Build history of the part. All positions in model axes, mm. A direction names the side the tool comes from. Give positions to 0.01 mm unless a question says otherwise; leave off trailing zeros. Write each loop counter-clockwise with the first axis right and the second up, starting at its lowest first coordinate (ties: lowest second). Pieces come first, ordered by that corner, then holes. Notation, with made-up numbers: (-11.5, 55) -> (25.5, 55) arc R19 cw to (25.5, 90) -> close; hole circle Ø5 at (-28, 74.5). An arc over 180 degrees is marked (long way). Put each result on its own line as item: value.
from build123d import *

# Parameters (mm, degrees)
SKETCH3_R           = 2.15
BOSS_EXTRUDE1_DEPTH = 5
SKETCH4_R           = 36
BOSS_EXTRUDE2_DEPTH = 41
SKETCH5_R           = 9.55
CUT_EXTRUDE1_DEPTH  = 6.2
SKETCH6_R           = 32
CUT_EXTRUDE2_DEPTH  = 36
SKETCH8_R           = 6
CUT_EXTRUDE3_DEPTH  = 76.060242472


with BuildPart() as part:
    # Sketch3 → Boss-Extrude1 (new body)
    with BuildSketch(Plane(origin=(0, 0, 0), x_dir=(1, 0, 0), z_dir=(0, 1, 0))):
        with BuildLine():
            Line((-35, 45), (35, 45))
            ThreePointArc((35, 45), (42.071067812, 42.071067812), (45, 35))
            Line((45, 35), (45, -35))
            ThreePointArc((45, -35), (42.071067812, -42.071067812), (35, -45))
            Line((35, -45), (-35, -45))
            ThreePointArc((-35, -45), (-42.071067812, -42.071067812), (-45, -35))
            Line((-45, -35), (-45, 35))
            ThreePointArc((-45, 35), (-42.071067812, 42.071067812), (-35, 45))
        make_face()
        with Locations(Location((-36, 36, 0), (0, 0, 270))):
            Circle(SKETCH3_R, mode=Mode.SUBTRACT)
        with Locations(Location((36, 36, 0), (0, 0, 270))):
            Circle(SKETCH3_R, mode=Mode.SUBTRACT)
        with Locations(Location((36, -36, 0), (0, 0, 270))):
            Circle(SKETCH3_R, mode=Mode.SUBTRACT)
        with Locations(Location((-36, -36, 0), (0, 0, 270))):
            Circle(SKETCH3_R, mode=Mode.SUBTRACT)
    extrude(amount=BOSS_EXTRUDE1_DEPTH)

    # Sketch4 → Boss-Extrude2 (add)
    with BuildSketch(Plane(origin=(0, 5, 0), x_dir=(1, 0, 0), z_dir=(0, 1, 0))):
        with Locations(Location((0, 0, 0), (0, 0, 270))):
            Circle(SKETCH4_R)
    extrude(amount=BOSS_EXTRUDE2_DEPTH)

    # Sketch5 → Cut-Extrude1 (cut)
    with BuildSketch(Plane(origin=(0, 46, 0), x_dir=(1, 0, 0), z_dir=(0, 1, 0))):
        with Locations(Location((0, 0, 0), (0, 0, 270))):
            Circle(SKETCH5_R)
    extrude(amount=-CUT_EXTRUDE1_DEPTH, mode=Mode.SUBTRACT)

    # Sketch6 → Cut-Extrude2 (cut)
    with BuildSketch(Plane.XZ):
        with Locations(Location((0, 0, 0), (0, 0, 270))):
            Circle(SKETCH6_R)
    extrude(amount=-CUT_EXTRUDE2_DEPTH, mode=Mode.SUBTRACT)

    # Sketch8 → Cut-Extrude3 (cut, through all)
    with BuildSketch(Plane(origin=(0, 39.8, 0), x_dir=(1, 0, 0), z_dir=(0, 1, 0))):
        with Locations(Location((0, 0, 0), (0, 0, 270))):
            Circle(SKETCH8_R)
    extrude(amount=-CUT_EXTRUDE3_DEPTH, mode=Mode.SUBTRACT)


solid = part.part
1) Pull direction Z, two halves, no side cores. Call faces 4 (the flat face through (31, 5, -21)), 5 (the flat face through (-6.2, 39.8, -0.1)), 6 (the flat face through (0, 2, -45)), 7 (the cylindrical face through (-41.99, 2.46, 42.15)): released by +Z, released by -Z, zero draft, split by the parting line, or undercut.
Filled sheet:
face 4: zero draft
face 5: undercut
face 6: released by -Z
face 7: released by +Z
2) Wall check: L1, parallel to X at y = 3, z = 36; L2, parallel to X at y = 16, z = 0; L3, parallel to Y at x = 19.5, z = -13. Give the ranges that are in metal, low to high.
Filled sheet:
L1: -44.95 to -38.15, -33.85 to 33.85, 38.15 to 44.95
L2: -36 to -32, 32 to 36
L3: 36 to 46
3) Slice it at D-D (y = 7.5). Write the cut outline in (x, z).
Filled sheet:
outline: circle Ø72 at (0, 0); hole circle Ø64 at (0, 0)
4) Slice it at C-C (x = -23.5). Write the cut outline in (y, z), plus the area to 3 significant figures.
Filled sheet:
outline: (0, -45) -> (5, -45) -> (5, -27.27) -> (46, -27.27) -> (46, 27.27) -> (5, 27.27) -> (5, 45) -> (0, 45) -> (0, 21.72) -> (36, 21.72) -> (36, -21.72) -> (0, -21.72) -> close
area: 1,120 mm2
5) Slice it at B-B (z = 0). Write the cut outline in (x, y), plus the area to 3 significant figures.
Filled sheet:
outline: (-45, 0) -> (-32, 0) -> (-32, 36) -> (-6, 36) -> (-6, 39.8) -> (-9.55, 39.8) -> (-9.55, 46) -> (-36, 46) -> (-36, 5) -> (-45, 5) -> close; (6, 36) -> (32, 36) -> (32, 0) -> (45, 0) -> (45, 5) -> (36, 5) -> (36, 46) -> (9.55, 46) -> (9.55, 39.8) -> (6, 39.8) -> close
area: 934 mm2
6) Slice it at A-A (x = 0). Write the cut outline in (y, z), plus the area to 3 significant figures.
Filled sheet:
outline: (0, -45) -> (5, -45) -> (5, -36) -> (46, -36) -> (46, -9.55) -> (39.8, -9.55) -> (39.8, -6) -> (36, -6) -> (36, -32) -> (0, -32) -> close; (0, 32) -> (36, 32) -> (36, 6) -> (39.8, 6) -> (39.8, 9.55) -> (46, 9.55) -> (46, 36) -> (5, 36) -> (5, 45) -> (0, 45) -> close
area: 934 mm2
7) Pin check, flat tips, straight feed: pin 1 (19 mm diameter, centred on x = -15.5, z = 14, fed in from -Y); pin 2 (6 mm diameter, centred on x = -11.5, y = 12, fed in from +Z); pin 3 (2 mm diameter, centred on x = -28.5, y = 29, fed in from -Z). Stop position of each tip, or through.
Filled sheet:
pin 1: y = 36
pin 2: z = 34.98
pin 3: z = -23.23
8) Tool access for faces 1 (the flat face through (-45, 2, 0)), 2 (the cylindrical face through (-31.24, 17.75, 6.94)), 3 (the cylindrical face through (2.9, 42.9, 9.1)): list every direction of +Z, -Z, +X, -X, +Y, -Y with a clear straight run to the whole face (end or side of a thin tool).
Filled sheet:
face 1: +Z, -Z, -X, +Y, -Y
face 2: -Y
face 3: +Y
